Build history of the part. All positions in model axes, mm. Face numbers are marked on the shaded views. Give positions to 0.01 mm unless a question says otherwise; leave off trailing zeros. Order: outer loops, then holes, each group sorted by start corner. A loop starts at its lowest first (then second) coordinate and runs counter-clockwise, first axis right, second up. Notation, with made-up numbers: (28.25, 47) - (82.25, 47) arc R22 ccw to (82.25, 65) - close; hole circle Ø9 at (29.5, -13). An arc over 180 degrees is marked (long way). One line per item, written item: value.
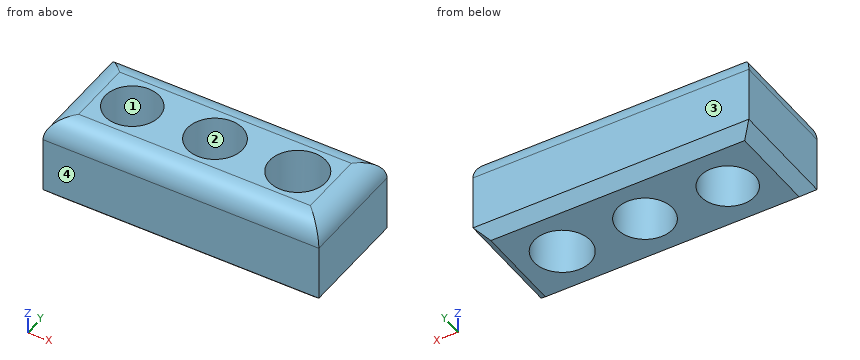
```python
from build123d import *

# Parameters (mm, degrees)
F0_W     = 25
F0_H     = 10
F0_R     = 2.45
F0_R_2   = 2.5
F0_R_3   = 2.55
F1_DEPTH = 8
F2_R     = 2
F3_SIZE  = 1


with BuildPart() as f1:
    # F0 (on Top) → F1 (new body)
    with BuildSketch(Plane.XY):
        Rectangle(F0_W, F0_H)
        with Locations((-7.5, 0)):
            Circle(F0_R, mode=Mode.SUBTRACT)
        Circle(F0_R_2, mode=Mode.SUBTRACT)
        with Locations((7.5, 0)):
            Circle(F0_R_3, mode=Mode.SUBTRACT)
    extrude(amount=F1_DEPTH)

    # F2
    f2_edges = [f1.edges().sort_by_distance(p)[0] for p in [
        (0, -5, 8),
        (-12.5, 0, 8),
        (0, 5, 8),
        (12.5, 0, 8),
    ]]
    fillet(f2_edges, radius=F2_R)

    # F3
    f3_edges = [f1.edges().sort_by_distance(p)[0] for p in [
        (-12.5, 0, 0),
        (0, -5, 0),
        (0, 5, 0),
        (12.5, 0, 0),
    ]]
    chamfer(f3_edges, length=F3_SIZE)


solid = f1.part
```
(1) Drill centre lines: line 1 (X direction, y = 0.25, z = 5.25); line 2 (Y direction, x = 0, z = 5.75); line 3 (X direction, y = 2, z = 2). Where is each one in solid material? Low to high.
Completed:
line 1: -12.5 to -9.94, -5.06 to -2.49, 2.49 to 4.96, 10.04 to 12.5
line 2: -5 to -2.5, 2.5 to 5
line 3: -12.5 to -8.92, -6.08 to -1.5, 1.5 to 5.92, 9.08 to 12.5
(2) Slice it at C-C, the plane z = 1.25. Give the cut face in (x, y), and give its area (3 significant figures).
Completed:
outline: (-12.5, -5) - (12.5, -5) - (12.5, 5) - (-12.5, 5) - close; hole circle Ø4.9 at (-7.5, 0); hole circle Ø5 at (0, 0); hole circle Ø5.1 at (7.5, 0)
area: 191 mm²
(3) Slice it at D-D, the plane x = 0. Give the cut face in (y, z), and give its area (3 significant figures).
Completed:
outline: (-5, 1) - (-4, 0) - (-2.5, 0) - (-2.5, 8) - (-3, 8) arc R2 ccw to (-5, 6) - close; (2.5, 0) - (4, 0) - (5, 1) - (5, 6) arc R2 ccw to (3, 8) - (2.5, 8) - close
area: 37.3 mm²
(4) Slice it at B-B, the plane y = 0. Give the cut face in (x, z).
Completed:
outline: (-12.5, 1) - (-11.5, 0) - (-9.95, 0) - (-9.95, 8) - (-10.5, 8) arc R2 ccw to (-12.5, 6) - close; (-5.05, 0) - (-2.5, 0) - (-2.5, 8) - (-5.05, 8) - close; (2.5, 0) - (4.95, 0) - (4.95, 8) - (2.5, 8) - close; (10.05, 0) - (11.5, 0) - (12.5, 1) - (12.5, 6) arc R2 ccw to (10.5, 8) - (10.05, 8) - close
(5) Pin check, flat tips, straight feed: P1, Ø3, axis at x = -7.5, y = 0, coming from the +Z side; P2, Ø5, axis at x = 8.5, y = -0.5, coming from the +Z side. Stop position of each tip, or through.
Completed:
P1: through
P2: z = 8
(6) Slice it at A-A, the plane x = -7.5. Give the cut face in (y, z), and give its area (3 significant figures).
Completed:
outline: (-5, 1) - (-4, 0) - (-2.45, 0) - (-2.45, 8) - (-3, 8) arc R2 ccw to (-5, 6) - close; (2.45, 0) - (4, 0) - (5, 1) - (5, 6) arc R2 ccw to (3, 8) - (2.45, 8) - close
area: 38.1 mm²
(7) Pull direction Y, two halves, no side cores. Call the marked faces 1, 2, 3 and 4: +Y half, -Y half, draft (parallel to the pull), parting line (faces both ways), or undercut.
Completed:
face 1: undercut
face 2: undercut
face 3: +Y half
face 4: -Y half
